Geometry check sheet. Reference: the model listing, model coordinates, mm. A direction names the side the tool comes from. Coordinates: 2 decimals unless noted, no trailing zeros. Loops run counter-clockwise (first coordinate to the right, second up) from the corner with the lowest first, then second, coordinate; pieces in that order, holes last. Notation, with made-up numbers: (61, 34) -> (109, 34) arc R4 ccw to (109, 40) -> close; hole circle Ø1 at (0.5, 75). An arc over 180 degrees is marked (long way). Answer as a JSON object with one key per item and string values.
from build123d import *

# Parameters (mm, degrees)
SKETCH2_R           = 2.1
SKETCH2_R_2         = 5.5
BOSS_EXTRUDE1_DEPTH = 1


with BuildPart() as part:
    # Sketch2 → Boss-Extrude1 (new body)
    with BuildSketch(Plane.XY):
        with BuildLine():
            Line((4.823205975, -0.488496739), (9.823205975, -0.488496739))
            ThreePointArc((9.823205975, -0.488496739), (12.6516331, 0.683076137), (13.823205975, 3.511503261))
            Line((13.823205975, 3.511503261), (13.823205975, 30.511503261))
            ThreePointArc((13.823205975, 30.511503261), (13.530312756, 31.218610043), (12.823205975, 31.511503261))
            Line((12.823205975, 31.511503261), (6.823205975, 31.511503261))
            ThreePointArc((6.823205975, 31.511503261), (6.116099194, 31.218610043), (5.823205975, 30.511503261))
            Line((5.823205975, 30.511503261), (5.823205975, 16.161503261))
            ThreePointArc((5.823205975, 16.161503261), (4.6516331, 13.333076137), (1.823205975, 12.161503261))
            Line((1.823205975, 12.161503261), (-9.176794025, 12.161503261))
            ThreePointArc((-9.176794025, 12.161503261), (-12.00522115, 10.989930386), (-13.176794025, 8.161503261))
            Line((-13.176794025, 8.161503261), (-13.176794025, -21.488496739))
            ThreePointArc((-13.176794025, -21.488496739), (-12.883900806, -22.19560352), (-12.176794025, -22.488496739))
            Line((-12.176794025, -22.488496739), (-0.176794025, -22.488496739))
            ThreePointArc((-0.176794025, -22.488496739), (0.530312756, -22.19560352), (0.823205975, -21.488496739))
            Line((0.823205975, -21.488496739), (0.823205975, -4.488496739))
            ThreePointArc((0.823205975, -4.488496739), (1.99477885, -1.660069614), (4.823205975, -0.488496739))
        make_face()
        with Locations((-10.376794025, -16.588496739)):
            Circle(SKETCH2_R, mode=Mode.SUBTRACT)
        with Locations((-10.376794025, -10.588496739)):
            Circle(SKETCH2_R, mode=Mode.SUBTRACT)
        with Locations((-6.526794025, 4.661503261)):
            Circle(SKETCH2_R_2, mode=Mode.SUBTRACT)
    extrude(amount=BOSS_EXTRUDE1_DEPTH)


solid = part.part
1. Section check A-A, the plane y = 5.5. Record the boundary of the cut face in (x, z).
Evaluation:
{"outline": "(-13.18, 0) -> (-11.96, 0) -> (-11.96, 1) -> (-13.18, 1) -> close; (-1.09, 0) -> (13.82, 0) -> (13.82, 1) -> (-1.09, 1) -> close"}
2. Section check C-C, the plane x = -5. Record the boundary of the cut face in (y, z).
Evaluation:
{"outline": "(-22.49, 0) -> (-0.62, 0) -> (-0.62, 1) -> (-22.49, 1) -> close; (9.95, 0) -> (12.16, 0) -> (12.16, 1) -> (9.95, 1) -> close"}
3. Section check B-B, the plane z = 0.65. Record the boundary of the cut face in (x, y).
Evaluation:
{"outline": "(-13.18, -21.49) arc R1 ccw to (-12.18, -22.49) -> (-0.18, -22.49) arc R1 ccw to (0.82, -21.49) -> (0.82, -4.49) arc R4 cw to (4.82, -0.49) -> (9.82, -0.49) arc R4 ccw to (13.82, 3.51) -> (13.82, 30.51) arc R1 ccw to (12.82, 31.51) -> (6.82, 31.51) arc R1 ccw to (5.82, 30.51) -> (5.82, 16.16) arc R4 cw to (1.82, 12.16) -> (-9.18, 12.16) arc R4 ccw to (-13.18, 8.16) -> close; hole circle Ø4.2 at (-10.38, -16.59); hole circle Ø4.2 at (-10.38, -10.59); hole circle Ø11 at (-6.53, 4.66)"}
4. Depth check by flat-ended pin: P1, Ø0.5, axis at y = 22, z = 0.5, coming from the -X side; P2, Ø10, axis at x = -6.53, y = 4.66, coming from the -Z side; P3, Ø0.5, axis at y = -14, z = 0.5, coming from the +X side; P4, Ø0.5, axis at x = 6, z = 0.5, coming from the -Y side. Enter the tip coordinate at first touch or a pass-through.
Evaluation:
{"P1": "stops at x = 5.82", "P2": "passes through", "P3": "stops at x = 0.82", "P4": "stops at y = -0.49"}
5. Mould release check, pull along Y, two halves, no side actions. Record for faces 4 (the face through (7.3, -0.488, 0.5)), 5 (the face through (13.823, 16.8, 0.5)), 6 (the face through (-11.925, -9.169, 0.493)): released by +Y, released by -Y, zero draft, split by the parting line, or undercut.
Evaluation:
{"face 4": "released by -Y", "face 5": "zero draft", "face 6": "undercut"}
6. Section check D-D, the plane y = 24. Record the boundary of the cut face in (x, z), then the cut area to 3 significant figures.
Evaluation:
{"outline": "(5.82, 0) -> (13.82, 0) -> (13.82, 1) -> (5.82, 1) -> close", "area": "8.00 mm^2"}
7. Thickness scan on probe 1 along X at (y, z) = (-10.5, 0.2); probe 2 along X at (y, z) = (22.5, 0.4); probe 3 along Y at (x, z) = (-10, 0.75). Record the ranges inside material, lowest first. Write a range as from..to.
Evaluation:
{"probe 1": "x = -13.18..-12.47, -8.28..0.82", "probe 2": "x = 5.82..13.82", "probe 3": "y = -22.49..-18.65, -14.52..-12.65, -8.52..0.4, 8.93..12.08"}
8. Tool access check on faces 1 (the face through (-13.177, -6.5, 0.5)), 2 (the face through (0.823, -13.1, 0.5)), 3 (the face through (5.823, 23.4, 0.5)). Record the directions out of +Z, -Z, +X, -X, +Y, -Y that give a thin tool (end or side, any length) a straight path to the whole face; none if there is none.
Evaluation:
{"face 1": "+Z, -Z, -X, +Y, -Y", "face 2": "+Z, -Z, +X, -Y", "face 3": "+Z, -Z, -X, +Y"}
